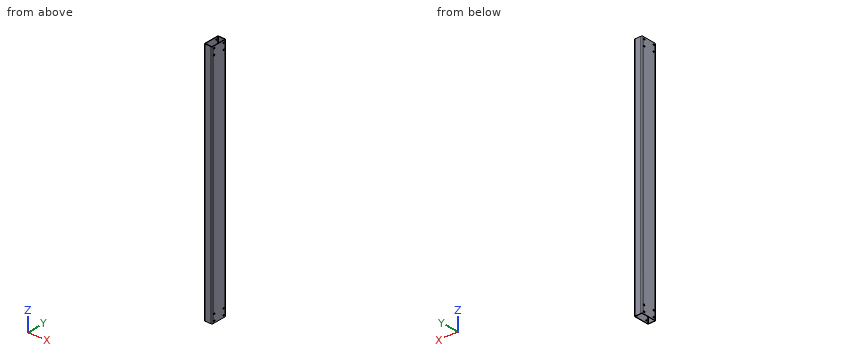
from build123d import *

# Parameters (mm, degrees)
BOSS_EXTRUDE1_DEPTH = 1220
SKETCH2_R           = 3.5
CUT_EXTRUDE1_DEPTH  = 41


with BuildPart() as part:
    # Sketch1 → Boss-Extrude1 (new body)
    with BuildSketch(Plane.XY):
        with BuildLine():
            Line((-15, -40), (15, -40))
            ThreePointArc((15, -40), (18.535533906, -38.535533906), (20, -35))
            Line((20, -35), (20, 35))
            ThreePointArc((20, 35), (18.535533906, 38.535533906), (15, 40))
            Line((15, 40), (-15, 40))
            ThreePointArc((-15, 40), (-18.535533906, 38.535533906), (-20, 35))
            Line((-20, 35), (-20, -35))
            ThreePointArc((-20, -35), (-18.535533906, -38.535533906), (-15, -40))
        make_face()
        with BuildLine():
            Line((-17.5, -35), (-17.5, 35))
            ThreePointArc((-17.5, 35), (-16.767766953, 36.767766953), (-15, 37.5))
            Line((-15, 37.5), (15, 37.5))
            ThreePointArc((15, 37.5), (16.767766953, 36.767766953), (17.5, 35))
            Line((17.5, 35), (17.5, -35))
            ThreePointArc((17.5, -35), (16.767766953, -36.767766953), (15, -37.5))
            Line((15, -37.5), (-15, -37.5))
            ThreePointArc((-15, -37.5), (-16.767766953, -36.767766953), (-17.5, -35))
        make_face(mode=Mode.SUBTRACT)
    extrude(amount=BOSS_EXTRUDE1_DEPTH)

    # Sketch2 → Cut-Extrude1 (cut, through all)
    with BuildSketch(Plane.ZY.offset(20)):
        with Locations((10.4, 27.5)):
            Circle(SKETCH2_R)
        with Locations((40.4, 27.5)):
            Circle(SKETCH2_R)
        with Locations((40.4, -27.5)):
            Circle(SKETCH2_R)
        with Locations((10.4, -27.5)):
            Circle(SKETCH2_R)
    cut_extrude1 = extrude(amount=-CUT_EXTRUDE1_DEPTH, mode=Mode.SUBTRACT)

    # Mirror1: Cut-Extrude1 across plane
    add(cut_extrude1.mirror(Plane.XY.offset(610)), mode=Mode.SUBTRACT)


solid = part.part
Geometry check sheet. Reference: the model listing, model coordinates, mm. Give positions to 0.01 mm unless a question says otherwise; leave off trailing zeros. Order: outer loops, then holes, each group sorted by start corner. A loop starts at its lowest first (then second) coordinate and runs counter-clockwise, first axis right, second up.
1. Depth check by flat-ended pin: pin 1 (5.5 mm diameter, centred on y = 27.5, z = 1209.6, fed in from -X). Enter the tip coordinate at first touch or a pass-through.
Completed:
pin 1: passes through
2. Scan lines: line 1 (Z direction, x = 19, y = -27); line 2 (Y direction, x = 8, z = 920); line 3 (X direction, y = -24, z = 973). Record each from-to range of solid material in increasing order.
Completed:
line 1: z = 0 to 6.94, 13.86 to 36.94, 43.86 to 1176.14, 1183.06 to 1206.14, 1213.06 to 1220
line 2: y = -40 to -37.5, 37.5 to 40
line 3: x = -20 to -17.5, 17.5 to 20
3. Sectioned sample at A-A (z = 171). Record the boundary of the cut face in (x, y).
Completed:
outline: (-20, -35) arc R5 ccw to (-15, -40) - (15, -40) arc R5 ccw to (20, -35) - (20, 35) arc R5 ccw to (15, 40) - (-15, 40) arc R5 ccw to (-20, 35) - close; hole (-17.5, -35) arc R2.5 ccw to (-15, -37.5) - (15, -37.5) arc R2.5 ccw to (17.5, -35) - (17.5, 35) arc R2.5 ccw to (15, 37.5) - (-15, 37.5) arc R2.5 ccw to (-17.5, 35) - close
4. Sectioned sample at B-B (y = -14). Record the boundary of the cut face in (x, z), then the cut area to 3 significant figures.
Completed:
outline: (-20, 0) - (-17.5, 0) - (-17.5, 1220) - (-20, 1220) - close; (17.5, 0) - (20, 0) - (20, 1220) - (17.5, 1220) - close
area: 6,100 mm2
